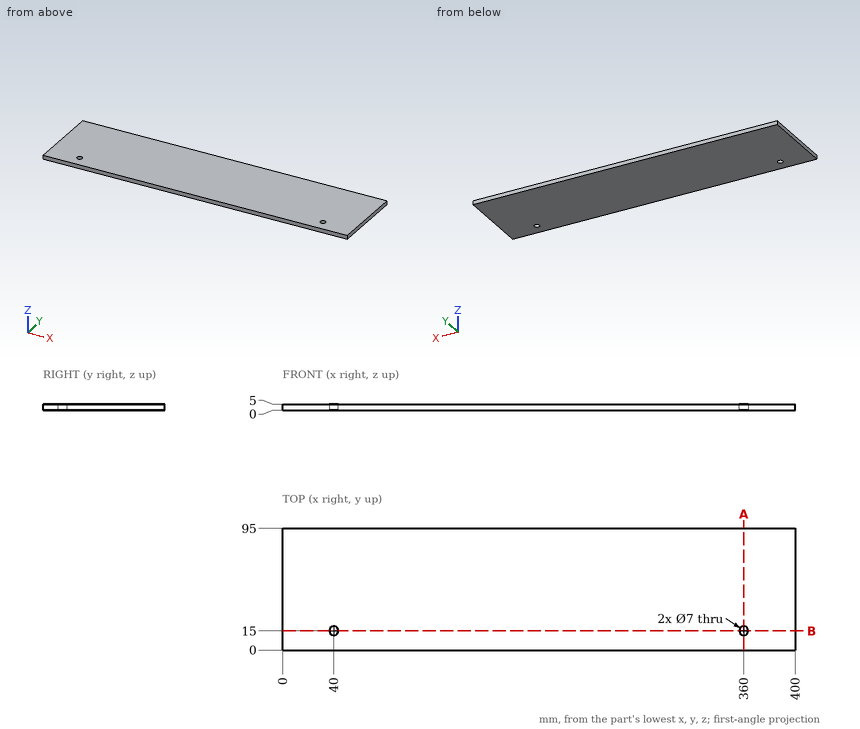
Part print with two shaded views. Sizes in mm from the minimum x, y, z corner. Round coordinates to 2 decimals unless told otherwise and drop trailing zeros. Loops run counter-clockwise (first coordinate to the right, second up) from the corner with the lowest first, then second, coordinate; pieces in that order, holes last. Notation, with made-up numbers: M -10.75,6.25 L 8.25,6.25 A21 ccw 8.25,32.25 Z; hole C -27.75,88 d8. An arc over 180 degrees is marked long. Return JSON: item names as keys, results as strings. Group by question number.
(1) Wall check: probe 1 along X at (y, z) = (15, 4.05); probe 2 along Y at (x, z) = (360, 1.4). Give the ranges that are in metal, low to high. Write a range as [from, to].
(2) Saw through at A-A, the plane x = 360. List the corners of the cut face in (y, z), and give its area (3 significant figures).
(3) Saw through at B-B, the plane y = 15. List the corners of the cut face in (x, z).
(4) Drop a flat-ended pin along its axis: P1, Ø6, axis at x = 345, y = 67, coming from the -Z side. Give the stop position or say it passes through.
Answer list:
{
 "1": {"probe 1": "[0, 36.5], [43.5, 356.5], [363.5, 400]", "probe 2": "[0, 11.5], [18.5, 95]"},
 "2": {"outline": "M 0,0 L 11.5,0 L 11.5,5 L 0,5 Z; M 18.5,0 L 95,0 L 95,5 L 18.5,5 Z", "area": "440 mm2"},
 "3": {"outline": "M 0,0 L 36.5,0 L 36.5,5 L 0,5 Z; M 43.5,0 L 356.5,0 L 356.5,5 L 43.5,5 Z; M 363.5,0 L 400,0 L 400,5 L 363.5,5 Z"},
 "4": {"P1": "z = 0"}
}
